Source: CAD feature listing. Evaluate the final solid. Frame: model axes, mm. Face numbers are marked on the shaded views. A direction names the side the tool comes from. Coordinates: 2 decimals unless noted, no trailing zeros. Order: outer loops, then holes, each group sorted by start corner. A loop starts at its lowest first (then second) coordinate and runs counter-clockwise, first axis right, second up.
```python
from build123d import *

# Parameters (mm, degrees)
KUGGLUCKA_DEPTH  = 12.8
CIRPATTERN_COUNT = 20
RITNING_4_R      = 3
AXELH_L_DEPTH    = 29.554110475


with BuildPart() as part:
    # Ritning 1 → Kugghjulsämne (revolve)
    with BuildSketch(Plane(origin=(0, 0, 0), x_dir=(0, 0, -1), z_dir=(1, 0, 0))):
        Polygon((6.4, 4.585), (6.4, 1.415), (14.2, 1.415), (14.2, -4.585), (6.4, -4.585), (-6.4, -4.585), (-6.4, 4.585), align=None)
    revolve(axis=Axis((0, -4.585, -14.2), (0, 0, 1)))

    # Ritning 2 → Kugglucka (cut)
    with BuildSketch(Plane.XY.offset(6.4)):
        with BuildLine():
            Line((1.302513782, 4.492023623), (1.302513782, 5.612023623))
            Line((1.302513782, 5.612023623), (-1.302513782, 5.612023623))
            Line((-1.302513782, 5.612023623), (-1.302513782, 4.492023623))
            ThreePointArc((-1.302513782, 4.492023623), (-1.099792064, 4.443429711), (-0.985557985, 4.269050704))
            ThreePointArc((-0.985557985, 4.269050704), (0, 3.465), (0.985557985, 4.269050704))
            ThreePointArc((0.985557985, 4.269050704), (1.099792064, 4.443429711), (1.302513782, 4.492023623))
        make_face()
    kugglucka = extrude(amount=-KUGGLUCKA_DEPTH, mode=Mode.SUBTRACT)

    # CirPattern: Kugglucka ×20 about axis
    cirpattern_axis = Axis((0, -4.585, 0), (0, 0, 1))
    for i in range(1, CIRPATTERN_COUNT):
        add(kugglucka.rotate(cirpattern_axis, i * 360 / CIRPATTERN_COUNT), mode=Mode.SUBTRACT)

    # Ritning 3 → Flänsar (revolve)
    with BuildSketch(Plane(origin=(0, 0, 0), x_dir=(0, 0, -1), z_dir=(1, 0, 0))):
        Polygon((-5.9, 3.0625), (-6.4, 3.0625), (-6.4, 4.585), (-6.988423234, 6.781025404), (-6.488423234, 6.915), (-5.9, 4.718974596), align=None)
        Polygon((5.9, 3.0625), (6.4, 3.0625), (6.4, 4.585), (6.988423234, 6.781025404), (6.488423234, 6.915), (5.9, 4.718974596), align=None)
    revolve(axis=Axis((0, -4.585, -6.4), (0, 0, 1)))

    # Ritning 4 → Axelhål (cut, through all)
    with BuildSketch(Plane.XY.offset(6.4)):
        with Locations((0, -4.585)):
            Circle(RITNING_4_R)
    extrude(amount=-AXELH_L_DEPTH, mode=Mode.SUBTRACT)


solid = part.part
```
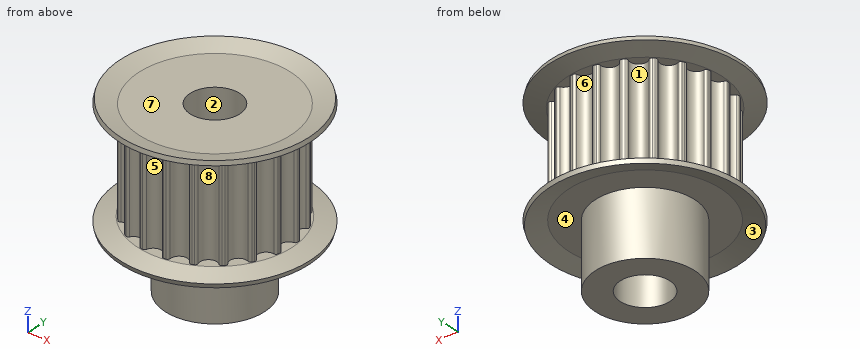
Q1. Set-up query: the marked faces 4, 5, 6, 7 and 8. Return all of +Z, -Z, +X, -X, +Y, -Y with unobstructed straight access to the full face (end or side cutting, diameter ignored); none if empty.
Solutions:
face 4: -Z
face 5: -Y
face 6: +Y
face 7: +Z
face 8: none
Q2. Pull-direction query (Z, two-part tool) for the marked faces 1, 2 and 3; classes: pulls with the +Z half, pulls with the -Z half, needs draft (parallel to the pull), parting line crosses it, or undercut.
Solutions:
face 1: undercut
face 2: needs draft
face 3: pulls with the -Z half
Q3. Section query A-A on x = 0. Output: boundary loops of the cut face in (y, z) (3 decimals).
Solutions:
outline: (-16.085, -6.488) - (-15.951, -6.988) - (-13.755, -6.4) - (-10.585, -6.4) - (-10.585, -14.2) - (-7.585, -14.2) - (-7.585, 6.4) - (-13.755, 6.4) - (-15.951, 6.988) - (-16.085, 6.488) - (-13.889, 5.9) - (-12.635, 5.9) - (-12.635, -5.9) - (-13.889, -5.9) - close; (-1.585, -14.2) - (1.415, -14.2) - (1.415, -6.4) - (4.585, -6.4) - (6.781, -6.988) - (6.915, -6.488) - (4.719, -5.9) - (3.465, -5.9) - (3.465, 5.9) - (4.719, 5.9) - (6.915, 6.488) - (6.781, 6.988) - (4.585, 6.4) - (-1.585, 6.4) - close
Q4. Pin query (flat end, axial travel): P1, Ø8, axis at x = 6, z = 1.5, coming from the +Y side; P2, Ø4, axis at x = 6, z = -11.5, coming from the +Y side; P3, Ø5, axis at x = -2, z = 3, coming from the -Y side. Return the tip coordinate at first contact, or that it passes through.
Solutions:
P1: stops at y = 3.67
P2: stops at y = -0.11
P3: stops at y = -13.66
Q5. Material intervals for line 1 along Z through (x, y) = (-2.5, -13); line 2 along Z through (x, y) = (3.5, 2); line 3 along X through (y, z) = (-11, -2.75), sorted ascending.
Solutions:
line 1: z = -6.4 to -5.9, 5.9 to 6.4
line 2: z = -6.4 to 6.4
line 3: x = -6.55 to -5.75, -4.9 to 4.9, 5.75 to 6.55
